Here's how the part is built. I have some questions about the finished solid (model axes, mm). A direction names the side the tool comes from. Round coordinates to 2 decimals unless told otherwise and drop trailing zeros. Write each loop counter-clockwise with the first axis right and the second up, starting at its lowest first coordinate (ties: lowest second). Pieces come first, ordered by that corner, then holes. Notation, with made-up numbers: (-26, -12) -> (12, -12) arc R34 ccw to (12, 21) -> close; hole circle Ø9 at (61.5, -30.75). An arc over 180 degrees is marked (long way). Answer as CSV lines item,"result".
```python
from build123d import *

# Parameters (mm, degrees)
SKETCH1_W           = 140
SKETCH1_H           = 70
SKETCH1_W_2         = 82
SKETCH1_H_2         = 42
BOSS_EXTRUDE1_DEPTH = 10
FILLET1_R           = 10
SKETCH2_R           = 2.75
CUT_EXTRUDE1_DEPTH  = 79.89866919
SKETCH3_R           = 4.125
CUT_EXTRUDE2_DEPTH  = 79.89866919
BOSS_EXTRUDE2_DEPTH = 10
FILLET2_R           = 5
SKETCH5_R           = 2.625
CUT_EXTRUDE3_DEPTH  = 79.89866919


with BuildPart() as part:
    # Sketch1 → Boss-Extrude1 (new body)
    with BuildSketch(Plane(origin=(0, 0, 0), x_dir=(1, 0, 0), z_dir=(0, 1, 0))):
        Rectangle(SKETCH1_W, SKETCH1_H)
        Rectangle(SKETCH1_W_2, SKETCH1_H_2, mode=Mode.SUBTRACT)
    extrude(amount=BOSS_EXTRUDE1_DEPTH)

    # Fillet1
    fillet1_edges = [part.edges().sort_by_distance(p)[0] for p in [
        (70, 5, 35),
        (-70, 5, 35),
        (-70, 5, -35),
        (70, 5, -35),
    ]]
    fillet(fillet1_edges, radius=FILLET1_R)

    # Sketch2 → Cut-Extrude1 (cut, through all)
    with BuildSketch(Plane(origin=(0, 10, 0), x_dir=(1, 0, 0), z_dir=(0, 1, 0))):
        with Locations(Location((-60, -25, 0), (0, 0, 270))):
            Circle(SKETCH2_R)
        with Locations(Location((-60, 25, 0), (0, 0, 90))):
            Circle(SKETCH2_R)
        with Locations(Location((60, -25, 0), (0, 0, 90))):
            Circle(SKETCH2_R)
        with Locations(Location((60, 25, 0), (0, 0, 270))):
            Circle(SKETCH2_R)
    extrude(amount=-CUT_EXTRUDE1_DEPTH, mode=Mode.SUBTRACT)

    # Sketch3 → Cut-Extrude2 (cut, through all)
    with BuildSketch(Plane(origin=(0, 10, 0), x_dir=(1, 0, 0), z_dir=(0, 1, 0))):
        with Locations(Location((-50, 0, 0), (0, 0, 270))):
            Circle(SKETCH3_R)
        with Locations(Location((50, 0, 0), (0, 0, 90))):
            Circle(SKETCH3_R)
    extrude(amount=-CUT_EXTRUDE2_DEPTH, mode=Mode.SUBTRACT)

    # Sketch4 → Boss-Extrude2 (add)
    with BuildSketch(Plane(origin=(0, 10, 0), x_dir=(1, 0, 0), z_dir=(0, 1, 0))):
        with BuildLine():
            Line((-41, 8.674675786), (-41, -8.674675786))
            ThreePointArc((-41, -8.674675786), (-37.5, 0), (-41, 8.674675786))
        make_face()
        with BuildLine():
            Line((41, 8.674675786), (41, -8.674675786))
            ThreePointArc((41, -8.674675786), (37.5, 0), (41, 8.674675786))
        make_face()
    extrude(amount=-BOSS_EXTRUDE2_DEPTH)

    # Fillet2
    fillet2_edges = [part.edges().sort_by_distance(p)[0] for p in [
        (41, 5, 21),
        (41, 5, -21),
        (-41, 5, -21),
        (-41, 5, 21),
    ]]
    fillet(fillet2_edges, radius=FILLET2_R)

    # Sketch5 → Cut-Extrude3 (cut, through all)
    with BuildSketch(Plane(origin=(0, 10, 0), x_dir=(1, 0, 0), z_dir=(0, 1, 0))):
        with Locations(Location((-61, 13, 0), (0, 0, 270))):
            Circle(SKETCH5_R)
        with Locations(Location((-61, -13, 0), (0, 0, 270))):
            Circle(SKETCH5_R)
        with Locations(Location((61, 13, 0), (0, 0, 270))):
            Circle(SKETCH5_R)
        with Locations(Location((61, -13, 0), (0, 0, 270))):
            Circle(SKETCH5_R)
    extrude(amount=-CUT_EXTRUDE3_DEPTH, mode=Mode.SUBTRACT)


solid = part.part
```
1. On a 3-axis mill with a long thin cutter (end or side, diameter ignored), from which of +Z, -Z, +X, -X, +Y, -Y can I reach the whole of each face in a straight line? I mean faces 1 (the face through (39, 5, 20)), 2 (the face through (-1, 10, -24)). Say none if no direction works.
Numbers:
face 1,"+Y, -Y"
face 2,"+Z, -Z, +X, -X, +Y"
2. Suppose I cut it at C-C on y = 8.5. Count the separate pieces of the cut face and the enclosed holes in it, and give its area (3 significant figures).
Numbers:
separate pieces,"1"
enclosed holes,"11"
area,"6,090 mm^2"
3. For pin 1 Ø1.5 at (y, z) = (5.5, -26.5) entering from +X, with a flat end and sliding along its axis, tell me the tip position at first contact or that it passes through.
Numbers:
pin 1,"stops at x = 69.97"
4. If we mould it in two halves opening along X, with no side actions, what happens to faces 3 (the face through (66.99, 5.07, -32.15)), 4 (the face through (-1, 5, -35)), 5 (the face through (-1, 5, 21))? For each: released by +X, released by -X, zero draft, split by the parting line, or undercut.
Numbers:
face 3,"released by +X"
face 4,"zero draft"
face 5,"undercut"
5. Suppose I cut it at A-A on x = 50. Please give me the cut outline in (y, z) (3 decimals), and give its area (4 significant figures).
Numbers:
outline,"(0, -35) -> (10, -35) -> (10, -4.125) -> (0, -4.125) -> close; (0, 4.125) -> (10, 4.125) -> (10, 35) -> (0, 35) -> close"
area,"617.5 mm^2"
6. Suppose I cut it at B-B on z = 13. Please give me the cut outline in (x, y) (3 decimals).
Numbers:
outline,"(-70, 0) -> (-63.625, 0) -> (-63.625, 10) -> (-70, 10) -> close; (-58.375, 0) -> (-41, 0) -> (-41, 10) -> (-58.375, 10) -> close; (41, 0) -> (58.375, 0) -> (58.375, 10) -> (41, 10) -> close; (63.625, 0) -> (70, 0) -> (70, 10) -> (63.625, 10) -> close"
7. Suppose I cut it at D-D on x = 25. Please give me the cut outline in (y, z), and give its area (3 significant figures).
Numbers:
outline,"(0, -35) -> (10, -35) -> (10, -21) -> (0, -21) -> close; (0, 21) -> (10, 21) -> (10, 35) -> (0, 35) -> close"
area,"280 mm^2"
8. If I drill on line 1 (X direction, y = 7.5, z = -13) (3 decimals); line 2 (Z direction, x = -34, y = 9); line 3 (X direction, y = 2.75, z = 25), over which ranges is the centre line in solid material (lowest first)?
Numbers:
line 1,"x = -70 to -63.625, -58.375 to -41, 41 to 58.375, 63.625 to 70"
line 2,"z = -35 to -21, 21 to 35"
line 3,"x = -70 to -62.75, -57.25 to 57.25, 62.75 to 70"
